The listing builds one solid part. Answer for the finished solid, in the listing's coordinates (mm). Coordinates: 2 decimals unless noted, no trailing zeros. Order: outer loops, then holes, each group sorted by start corner. A loop starts at its lowest first (then second) coordinate and runs counter-clockwise, first axis right, second up. Notation, with made-up numbers: (-2.75, -33.75) -> (13.25, -33.75) arc R19 cw to (13.25, -20.75) -> close; hole circle Ø7 at (7.5, 64.25). An arc over 180 degrees is marked (long way). Put each result on its own line as item: value. Start each with the question number.
```python
from build123d import *

# Parameters (mm, degrees)
F0_W     = 2000
F0_H     = 1750
F0_W_2   = 952
F0_H_2   = 32
F0_W_3   = 32
F0_H_3   = 827
F1_DEPTH = 33


with BuildPart() as f1:
    # F0 (on Front) → F1 (new body)
    with BuildSketch(Plane.XZ):
        with Locations((1000, 875)):
            Rectangle(F0_W, F0_H)
        Polygon((984, 32), (32, 32), (32, 859), (32, 891), (32, 1718), (984, 1718), (1016, 1718), (1968, 1718), (1968, 891), (1968, 859), (1968, 32), (1016, 32), align=None, mode=Mode.SUBTRACT)
        with Locations((508, 875)):
            Rectangle(F0_W_2, F0_H_2)
        with Locations((1000, 445.5)):
            Rectangle(F0_W_3, F0_H_3)
        with Locations((1000, 875)):
            Rectangle(F0_W_3, F0_H_2)
        with Locations((1000, 1304.5)):
            Rectangle(F0_W_3, F0_H_3)
        with Locations((1492, 875)):
            Rectangle(F0_W_2, F0_H_2)
    extrude(amount=F1_DEPTH)


solid = f1.part
```
(1) Find the intervals of material crossed by L1, parallel to Z at x = 1641, y = -19; L2, parallel to X at y = -12, z = 1002, in increasing order.
(2) The part is cut by section B-B on x = 520.5. Determine the outline of the cut face in (y, z), plus the area to 3 significant figures.
(3) The part is cut by section C-C on z = 1119. Determine the outline of the cut face in (x, y).
(4) The part is cut by section A-A on y = -22. Determine the outline of the cut face in (x, z), plus the area to 3 significant figures.
Worked out:
1. L1: 0 to 32, 859 to 891, 1718 to 1750
1. L2: 0 to 32, 984 to 1016, 1968 to 2000
2. outline: (-33, 0) -> (0, 0) -> (0, 32) -> (-33, 32) -> close; (-33, 859) -> (0, 859) -> (0, 891) -> (-33, 891) -> close; (-33, 1718) -> (0, 1718) -> (0, 1750) -> (-33, 1750) -> close
2. area: 3,170 mm2
3. outline: (0, -33) -> (32, -33) -> (32, 0) -> (0, 0) -> close; (984, -33) -> (1016, -33) -> (1016, 0) -> (984, 0) -> close; (1968, -33) -> (2000, -33) -> (2000, 0) -> (1968, 0) -> close
4. outline: (0, 0) -> (2000, 0) -> (2000, 1750) -> (0, 1750) -> close; hole (32, 32) -> (984, 32) -> (984, 859) -> (32, 859) -> close; hole (32, 891) -> (984, 891) -> (984, 1718) -> (32, 1718) -> close; hole (1016, 32) -> (1968, 32) -> (1968, 859) -> (1016, 859) -> close; hole (1016, 891) -> (1968, 891) -> (1968, 1718) -> (1016, 1718) -> close
4. area: 351,000 mm2
